Input: dimensioned drawing with shaded views. Units: mm. Origin: part minimum x, y, z. A direction names the side the tool comes from. Coordinates: 2 decimals unless noted, no trailing zeros. Order: outer loops, then holes, each group sorted by start corner. A loop starts at its lowest first (then second) coordinate and runs counter-clockwise, first axis right, second up.
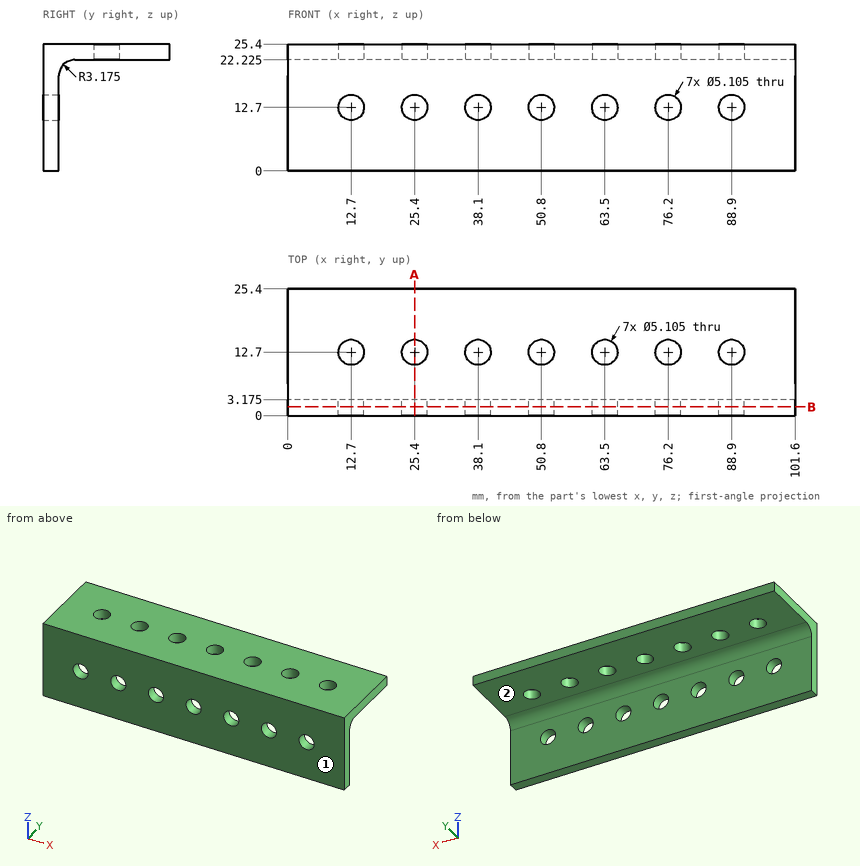
1. Access query for the marked faces 1 and 2. Directions: +Z, -Z, +X, -X, +Y, -Y. A direction counts if a zero-diameter tool reaches every point of the face in a straight line with its end or side. Return the directions, or none.
Findings:
face 1: +Z, -Z, +X, -X, -Y
face 2: -Z, +X, -X, +Y
2. Section query B-B on y = 1.75. Return loops of the section in (x, z) (1 decimal).
Findings:
outline: (0, 0) - (101.6, 0) - (101.6, 25.4) - (0, 25.4) - close; hole circle Ø5.1 at (12.7, 12.7); hole circle Ø5.1 at (25.4, 12.7); hole circle Ø5.1 at (38.1, 12.7); hole circle Ø5.1 at (50.8, 12.7); hole circle Ø5.1 at (63.5, 12.7); hole circle Ø5.1 at (76.2, 12.7); hole circle Ø5.1 at (88.9, 12.7)
3. Section query A-A on x = 25.4. Count the separate pieces of the cut face and the enclosed holes in it, plus the area to 3 significant figures.
Findings:
separate pieces: 3
enclosed holes: 0
area: 121 mm2
4. Ray query, line 1 (Z direction, x = 63.5, y = 2.75); line 2 (Z direction, x = 83, y = 11.25) (1 decimal). Return the intervals inside material, ascending.
Findings:
line 1: z = 0 to 10.15, 15.25 to 25.4
line 2: z = 22.2 to 25.4
5. Pin query (flat end, axial travel): P1, Ø2, axis at x = 83, y = 11, coming from the -Z side (3 decimals); P2, Ø4, axis at y = 4, z = 3.5, coming from the +X side; P3, Ø4, axis at x = 75.5, z = 5, coming from the +Y side (3 decimals); P4, Ø8, axis at x = 81, z = 16, coming from the +Y side. Return the tip coordinate at first contact, or that it passes through.
Findings:
P1: stops at z = 22.225
P2: stops at x = 101.6
P3: stops at y = 3.175
P4: stops at y = 3.32
